Could you check a few things on this model? Use its own coordinates, in mm. Face numbers are marked on the shaded views. A direction names the side the tool comes from. Round coordinates to 2 decimals unless told otherwise and drop trailing zeros. Loops run counter-clockwise (first coordinate to the right, second up) from the corner with the lowest first, then second, coordinate; pieces in that order, holes last. Notation, with made-up numbers: M -30,2.5 L -24,2.5 A25 ccw -24,33.5 Z; hole C 9,38.5 d7. An arc over 180 degrees is marked long. Answer in a Markdown table with one row per item.
```python
from build123d import *

# Parameters (mm, degrees)
SKETCH4_R           = 8
SKETCH4_R_2         = 3.96875
SKETCH4_R_3         = 2
SKETCH4_R_4         = 1.89865
BOSS_EXTRUDE2_DEPTH = 6.35
BOSS_EXTRUDE5_START = -3.5
SKETCH31_R          = 8
SKETCH31_R_2        = 6.025
BOSS_EXTRUDE5_DEPTH = 3.5


with BuildPart() as part:
    # Sketch4 → Boss-Extrude2 (new body)
    with BuildSketch(Plane(origin=(0, 0, 0), x_dir=(1, 0, 0), z_dir=(0, 1, 0))):
        with BuildLine():
            Line((40.257702493, -18.4375), (22.483900583, -18.4375))
            ThreePointArc((22.483900583, -18.4375), (21.500464498, -18.308390309), (20.583679925, -17.929811531))
            Line((20.583679925, -17.929811531), (10.779476649, -12.288263354))
            ThreePointArc((10.779476649, -12.288263354), (9.307944036, -11.804768953), (7.765559219, -11.946980575))
            Line((7.765559219, -11.946980575), (-16.517810325, -19.369406885))
            ThreePointArc((-16.517810325, -19.369406885), (-20.348558836, -18.710969534), (-22.098, -15.24))
            Line((-22.098, -15.24), (-22.098, 4.987500122))
            ThreePointArc((-22.098, 4.987500122), (-20.982076836, 7.681576958), (-18.288, 8.797500122))
            Line((-18.288, 8.797500122), (-12.3825, 8.797500122))
            ThreePointArc((-12.3825, 8.797500122), (-9.688423164, 9.913423286), (-8.5725, 12.607500122))
            Line((-8.5725, 12.607500122), (-8.5725, 26.9875))
            ThreePointArc((-8.5725, 26.9875), (-7.456576836, 29.681576836), (-4.7625, 30.7975))
            Line((-4.7625, 30.7975), (52.3875, 30.7975))
            ThreePointArc((52.3875, 30.7975), (55.081576836, 29.681576836), (56.1975, 26.9875))
            Line((56.1975, 26.9875), (56.1975, 19.362095927))
            ThreePointArc((56.1975, 19.362095927), (55.797199918, 17.662082259), (54.680415238, 16.319294633))
            Line((54.680415238, 16.319294633), (48.985566477, 12.027918285))
            ThreePointArc((48.985566477, 12.027918285), (47.868781798, 10.685130659), (47.468481715, 8.985116992))
            Line((47.468481715, 8.985116992), (47.468481715, -10.980610773))
            ThreePointArc((47.468481715, -10.980610773), (47.203372649, -12.376980446), (46.444939319, -13.579024524))
            Line((46.444939319, -13.579024524), (43.044160097, -17.225913752))
            ThreePointArc((43.044160097, -17.225913752), (41.776936446, -18.121498883), (40.257702493, -18.4375))
        make_face()
        with Locations(Location((0, 0, 0), (0, 0, 270))):
            Circle(SKETCH4_R, mode=Mode.SUBTRACT)
        with Locations(Location((-1.5875, 21.9075, 0), (0, 0, 270))):
            Circle(SKETCH4_R_2, mode=Mode.SUBTRACT)
        with Locations(Location((49.2125, 21.9075, 0), (0, 0, 270))):
            Circle(SKETCH4_R_2, mode=Mode.SUBTRACT)
        with Locations(Location((24.012521227, -14.703599027, 0), (0, 0, 270))):
            Circle(SKETCH4_R_3, mode=Mode.SUBTRACT)
        with Locations(Location((-17.78, -15.24, 0), (0, 0, 270))):
            Circle(SKETCH4_R_3, mode=Mode.SUBTRACT)
        with Locations(Location((18.000000004, 0, 0), (0, 0, 270))):
            Circle(SKETCH4_R_4, mode=Mode.SUBTRACT)
        with Locations(Location((-18.000000004, 0, 0), (0, 0, 270))):
            Circle(SKETCH4_R_4, mode=Mode.SUBTRACT)
    extrude(amount=-BOSS_EXTRUDE2_DEPTH)

    # Sketch31 → Boss-Extrude5 (add)
    with BuildSketch(Plane.XZ.offset(6.35).offset(BOSS_EXTRUDE5_START)):
        with Locations(Location((0, 0, 0), (0, 0, 90))):
            Circle(SKETCH31_R)
        with Locations(Location((0, 0, 0), (0, 0, 270))):
            Circle(SKETCH31_R_2, mode=Mode.SUBTRACT)
    extrude(amount=BOSS_EXTRUDE5_DEPTH)


solid = part.part
```
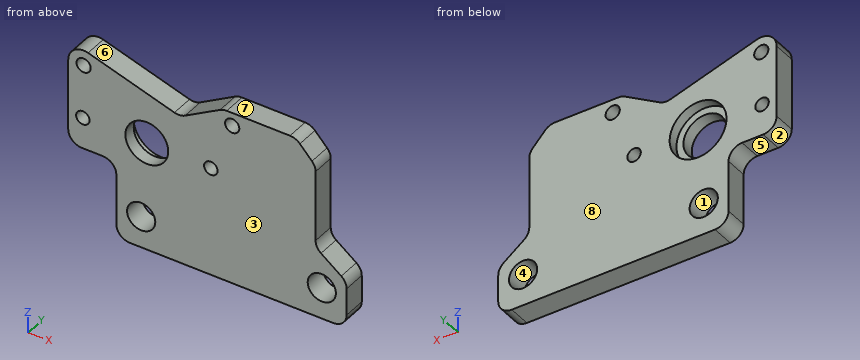
1) I want a section at B-B, the plane z = -23.5. Please give me the cut outline in (x, y), plus the area to 3 significant figures.
Computed:
| item | result |
|---|---|
| outline | M -8.57,-6.35 L -5.22,-6.35 L -5.22,0 L -8.57,0 Z; M 2.05,-6.35 L 45.58,-6.35 L 45.58,0 L 2.05,0 Z; M 52.85,-6.35 L 56.2,-6.35 L 56.2,0 L 52.85,0 Z |
| area | 319 mm² |
2) I want a section at A-A, the plane z = 0. Please give me the cut outline in (x, y) (3 decimals), plus the area to 3 significant figures.
Computed:
| item | result |
|---|---|
| outline | M -22.098,-6.35 L -19.899,-6.35 L -19.899,0 L -22.098,0 Z; M -16.101,-6.35 L -6.025,-6.35 L -6.025,-2.85 L -8,-2.85 L -8,0 L -16.101,0 Z; M 6.025,-6.35 L 16.101,-6.35 L 16.101,0 L 8,0 L 8,-2.85 L 6.025,-2.85 Z; M 19.899,-6.35 L 47.468,-6.35 L 47.468,0 L 19.899,0 Z |
| area | 306 mm² |
3) I want a section at D-D, the plane x = 51. Please give me the cut outline in (y, z).
Computed:
| item | result |
|---|---|
| outline | M -6.35,-30.8 L 0,-30.8 L 0,-25.45 L -6.35,-25.45 Z; M -6.35,-18.36 L 0,-18.36 L 0,-13.55 L -6.35,-13.55 Z |
4) Which directions (+Z, -Z, +X, -X, +Y, -Y) give clear straight access to the entire face, cutting with the end or side of a thin tool? Please do the marked faces 4, 5, 6, 7 and 8.
Computed:
| item | result |
|---|---|
| face 4 | +Y, -Y |
| face 5 | -Z, -X, +Y, -Y |
| face 6 | +Z, +Y, -Y |
| face 7 | +Z, +X, +Y, -Y |
| face 8 | +Z, -Z, +X, -X, +Y |
5) If we mould it in two halves opening along X, with no side actions, what happens to the marked faces 1, 2 and 3? For each: released by +X, released by -X, zero draft, split by the parting line, or undercut.
Computed:
| item | result |
|---|---|
| face 1 | undercut |
| face 2 | released by -X |
| face 3 | zero draft |
6) I want a section at C-C, the plane x = 0. State how many separate pieces and enclosed holes the cut face has, plus the area to 3 significant figures.
Computed:
| item | result |
|---|---|
| separate pieces | 3 |
| enclosed holes | 0 |
| area | 153 mm² |
7) I need wall thicknesses on line 1 (X direction, y = -1.15, z = 0); line 2 (X direction, y = -4.25, z = 0) (3 decimals); line 3 (Z direction, x = -18, y = -1.75). Which ranges of each line are inside material? Lowest first, please.
Computed:
| item | result |
|---|---|
| line 1 | x = -22.1 to -19.9, -16.1 to -8, 8 to 16.1, 19.9 to 47.47 |
| line 2 | x = -22.098 to -19.899, -16.101 to -6.025, 6.025 to 16.101, 19.899 to 47.468 |
| line 3 | z = -8.8 to -1.9, 1.9 to 13.25, 17.23 to 19.55 |
8) Will these pins go through, and if not, where does the flat tip stop? P1, Ø3.5, axis at x = 18, z = 0, coming from the +Y side; P2, Ø3, axis at y = -1, z = -8, coming from the -X side; P3, Ø3, axis at y = -4, z = -16, coming from the -X side.
Computed:
| item | result |
|---|---|
| P1 | passes through |
| P2 | stops at x = -21.78 |
| P3 | stops at x = -8.57 |
